Verification items for the finished model (mm, model axes). Coordinates: 2 decimals unless noted, no trailing zeros. Write each loop counter-clockwise with the first axis right and the second up, starting at its lowest first coordinate (ties: lowest second). Pieces come first, ordered by that corner, then holes. Notation, with made-up numbers: (-21.75, -7) -> (16.25, -7) arc R14 ccw to (16.25, 2) -> close; hole circle Ø1 at (63.5, -18). An arc over 180 degrees is marked (long way). Answer in a Markdown table with one row per item.
Solid Edge part; units mm, degrees
sketch "Sketch1" plane through (0, 0, 0) normal (0, -1, 0) x (1, 0, 0)
  line L0 (-10, -4) -> (10, -4)
  arc A0 (10, -4) -> (10, 4) centre (10, 0) ccw
  line L1 (10, 4) -> (-10, 4)
  arc A1 (-10, -4) -> (-10, 4) centre (-10, 0) cw
  dimension "D1" = 10
  dimension "D2" = 10
extrude "Ajout_matière_1" add sketch "Sketch1" along normal blind 3
sketch "Sketch2" plane through (0, -3, 0) normal (0, -1, 0) x (-1, 0, 0)
  circle A0 centre (-10, 0) radius 1.075
  circle A1 centre (10, 0) radius 1.075
extrude "Enlèvement_matière_1" cut sketch "Sketch2" against normal blind 5.6361
properties part number "12" material "MDF 3mm"
1. Section check D-D, the plane z = 3.75. Record the boundary of the cut face in (x, y), plus the area to 3 significant figures.
Geometry says:
| item | result |
|---|---|
| outline | (-11.39, -3) -> (11.39, -3) -> (11.39, 0) -> (-11.39, 0) -> close |
| area | 68.4 mm^2 |
2. Section check A-A, the plane z = 0. Record the boundary of the cut face in (x, y) (3 decimals).
Geometry says:
| item | result |
|---|---|
| outline | (-14, -3) -> (-11.075, -3) -> (-11.075, 0) -> (-14, 0) -> close; (-8.925, -3) -> (8.925, -3) -> (8.925, 0) -> (-8.925, 0) -> close; (11.075, -3) -> (14, -3) -> (14, 0) -> (11.075, 0) -> close |
3. Thickness scan on line 1 (X direction, y = -2.3, z = 0) (3 decimals); line 2 (Z direction, x = -10, y = -0.9) (3 decimals); line 3 (X direction, y = -2, z = 0.5). Record the ranges inside material, lowest first. Write a range as from..to.
Geometry says:
| item | result |
|---|---|
| line 1 | -14..-11.075, -8.925..8.925, 11.075..14 |
| line 2 | -4..-1.075, 1.075..4 |
| line 3 | -13.97..-10.95, -9.05..9.05, 10.95..13.97 |
4. Section check C-C, the plane x = 9.5. Record the boundary of the cut face in (y, z).
Geometry says:
| item | result |
|---|---|
| outline | (-3, -4) -> (0, -4) -> (0, -0.95) -> (-3, -0.95) -> close; (-3, 0.95) -> (0, 0.95) -> (0, 4) -> (-3, 4) -> close |
5. Section check B-B, the plane y = -2.2. Record the boundary of the cut face in (x, z) (3 decimals).
Geometry says:
| item | result |
|---|---|
| outline | (-10, -4) -> (10, -4) arc R4 ccw to (10, 4) -> (-10, 4) arc R4 ccw to start; hole circle Ø2.15 at (-10, 0); hole circle Ø2.15 at (10, 0) |
6. Mould release check, pull along Z, two halves, no side actions. Record for faces 1 (the cylindrical face through (-14, -1, 0)), 2 (the flat face through (0, -1, -4)), 3 (the cylindrical face through (11.074, -1.521, -0.047)), 4 (the flat face through (0, -3, 0)): released by +Z, released by -Z, zero draft, split by the parting line, or undercut.
Geometry says:
| item | result |
|---|---|
| face 1 | split by the parting line |
| face 2 | released by -Z |
| face 3 | undercut |
| face 4 | zero draft |
